from build123d import *

# Parameters (mm, degrees)
F1_DEPTH = 101.6
F1_TAPER = 7.556054046


with BuildPart() as f1:
    # F0 (on Top) → F1 (new body)
    with BuildSketch(Plane.XY):
        Polygon((0, 0), (-0.9788434916, 55.6218195157), (-35.4148902231, 0), align=None)
    extrude(amount=F1_DEPTH, taper=F1_TAPER)

    # F2: F1 across face


with BuildPart() as f1_1:
    add(f1.part)
    add(f1.part.mirror(Plane(origin=(-16.4023206536, 22.737179725, 31.6369417684), x_dir=(-0.5263932023, -0.8502412579, 0), z_dir=(-0.8428583491, 0.5218223667, 0.1314960875))))

    # F3: F1 across face


with BuildPart() as f1_2:
    add(f1_1.part)
    add(f1_1.part.mirror(Plane(origin=(-4.5973572795, 22.7371792838, 31.6369418981), x_dir=(-0.0175954682, 0.9998451878, 0), z_dir=(0.9911632216, 0.0174426813, 0.1314960875))))

    # F4: F1 across face


with BuildPart() as f1_3:
    add(f1_2.part)
    add(f1_2.part.mirror(Plane(origin=(10.5439699338, 33.6829824787, 38.4876798223), x_dir=(-0.9642022, 0.2651680929, 0), z_dir=(0.2399623244, 0.8725491765, 0.425530278))))

    # F5: F1 across face


with BuildPart() as f1_4:
    add(f1_3.part)
    add(f1_3.part.mirror(Plane(origin=(-21.3700903424, 33.1213526999, 34.2536909371), x_dir=(-0.9178751297, -0.3968693062, 0), z_dir=(-0.3726102349, 0.8617690066, 0.3442612266))))

    # F6: F1 across face


with BuildPart() as f1_5:
    add(f1_4.part)
    add(f1_4.part.mirror(Plane(origin=(-16.0760387074, 4.1965743618, 31.6369428308), x_dir=(1, 0, 0), z_dir=(0, -0.9913166895, 0.1314960875))))

    # F7: F1 across face


with BuildPart() as f1_6:
    add(f1_5.part)
    add(f1_5.part.mirror(Plane(origin=(22.2597853072, -4.1764689394, 44.1816075195), x_dir=(-0.5858563278, 0.8104149327, 0), z_dir=(0.7608774319, 0.5500452178, 0.3442612266))))

    # F8: F1 across face


with BuildPart() as f1_7:
    add(f1_6.part)
    add(f1_6.part.mirror(Plane(origin=(35.6016618602, 44.3371609674, 67.8410401107), x_dir=(-0.9178751298, -0.3968693062, 0), z_dir=(-0.3726102349, 0.8617690066, 0.3442612266))))

    # F9: F1 across face


with BuildPart() as f1_8:
    add(f1_7.part)
    add(f1_7.part.mirror(Plane(origin=(-53.5658558506, 42.7679738217, 56.0113238164), x_dir=(0.9642022, -0.265168093, 0), z_dir=(-0.2399623245, -0.8725491764, -0.425530278))))

    # F10: F1 across face


with BuildPart() as f1_9:
    add(f1_8.part)
    add(f1_8.part.mirror(Plane(origin=(-67.6744000884, -17.254319617, 81.3366041914), x_dir=(0.950172763, 0.3117237888, 0), z_dir=(0.2399623244, -0.7314349209, 0.638295417))))

    # F11: F1 across face


with BuildPart() as f1_10:
    add(f1_9.part)
    add(f1_9.part.mirror(Plane(origin=(-47.8862406141, 9.6288854157, 148.2567814243), x_dir=(-0.5016862394, -0.8650496617, 0), z_dir=(-0.7608774318, 0.4412714719, -0.4757573141))))

    # F12: F1 across face


with BuildPart() as f1_11:
    add(f1_10.part)
    add(f1_10.part.mirror(Plane(origin=(11.1666679236, 62.2499398733, 127.2140978003), x_dir=(0.3283942647, -0.9445407386, 0), z_dir=(-0.6028960247, -0.2096125541, 0.7697915046))))


solid = f1_11.part
Can you work these out from the model? Positions are in its coordinate system, mm. Give positions to 0.01 mm unless a question says otherwise; leave off trailing zeros. Order: outer loops, then holes, each group sorted by start corner. A loop starts at its lowest first (then second) coordinate and runs counter-clockwise, first axis right, second up. Notation, with made-up numbers: M -35,71 L 11,71 A15 ccw 11,87 Z; hole C -22,54.25 d6. An arc over 180 degrees is marked long. Use one line per item in the form item = value. Start each with the question number.
Item 1: If we section it at A-A (z = 44.5): Write out the boundary of the cut face in (x, y), then the cut area to 3 significant figures.
Item 2: Will these pins go through, and if not, where does the flat tip stop? pin 1 Ø4 at (y, z) = (45, 89.5) entering from +X; pin 2 Ø1.5 at (x, y) = (6.5, 15) entering from +Z; pin 3 Ø4 at (y, z) = (58, 38.5) entering from -X.
Item 3: If I drill on line 1 along Y through (x, z) = (-82, 75); line 2 along X through (y, z) = (-12.5, 106); line 3 along Z through (x, y) = (-0.5, -66), over which ranges is the centre line in solid material (lowest first)?
Item 4: If we section it at B-B (x = 14): Write out the boundary of the cut face in (y, z), then the cut area to 3 significant figures.
Item 5: If we section it at C-C (x = -56.5): Write out the boundary of the cut face in (y, z), then the cut area to 3 significant figures.
Outcome:
q1.outline = M -98.19,5.9 L -96.57,-3.49 L -90.31,-17.22 L -67.49,-49.34 L -62.1,-54.32 L -52.19,-59.29 L -27.7,-67.43 L -4.69,-68.9 L 14.39,-64.48 L 38.47,-50.99 L 48.93,-41.27 L 70.51,-4.06 L 73.95,5.9 L 73.57,13.42 L 63.9,40.06 L 54.14,61.68 L 50.05,66.63 L 24.46,85.5 L 8.47,91.25 L -7.59,95.66 L -15.24,95.08 L -44.29,87.68 L -63.89,76.04 L -81.86,56.16 L -88.01,43.75 L -97.07,17.05 Z
q1.area = 21,100 mm2
q2.pin_1 = 77.89
q2.pin_2 = 189.33
q2.pin_3 = -77.64
q3.line_1 = -50.16 to 77.32
q3.line_2 = -104.13 to 79.44
q3.line_3 = 40.47 to 147.69
q4.outline = M -79.45,90.85 L -74.3,64.83 L -64.21,43.74 L -52.67,25.89 L -44.87,18.99 L -30.29,12.26 L 0.5,3.78 L 32.44,3.93 L 48.27,6.63 L 57.6,11.27 L 73.39,25.49 L 88.63,43.22 L 100.39,66.99 L 105.23,86.24 L 104.94,103.05 L 97.47,130.75 L 94.09,138.1 L 77.86,159.63 L 58.77,174.38 L 33.1,185.38 L 24.9,187.73 L 16.38,187.6 L -11.28,183.67 L -33.55,174.41 L -54.83,157.86 L -60.01,151.64 L -74.44,126.84 L -79.11,110.69 Z
q4.area = 26,600 mm2
q5.outline = M -78.09,101.04 L -77.97,94.42 L -75.03,83.51 L -55.99,42.02 L -52.24,37.05 L -41.25,28.56 L -23.51,17.59 L 1.39,10.45 L 27.28,10.85 L 47.27,16.81 L 60.09,22.14 L 65.01,25.97 L 94.21,61.06 L 99.89,70.83 L 101.73,77.19 L 101.87,85.01 L 97.58,106.62 L 90.16,130.27 L 76.69,151.1 L 60.1,165.78 L 29.1,180.1 L 24.07,181.48 L 18.86,181.46 L -14.8,175.71 L -34.64,165.86 L -53.08,149.27 L -66.41,128.38 L -76.18,108.62 Z
q5.area = 23,100 mm2
